from build123d import *

# Parameters (mm, degrees)
SKETCH1_W           = 100
SKETCH1_H           = 70
BOSS_EXTRUDE1_DEPTH = 6.5
SKETCH2_R           = 11.5
CUT_EXTRUDE1_DEPTH  = 19
CUT_EXTRUDE2_DEPTH  = 8
FILLET1_R           = 10


with BuildPart() as part:
    # Sketch1 → Boss-Extrude1 (new body)
    with BuildSketch(Plane(origin=(0, 0, 0), x_dir=(1, 0, 0), z_dir=(0, 1, 0))):
        Rectangle(SKETCH1_W, SKETCH1_H)
    extrude(amount=BOSS_EXTRUDE1_DEPTH)

    # Sketch2 → Cut-Extrude1 (cut)
    with BuildSketch(Plane(origin=(10.212212675, 6.5, 1.842409503), x_dir=(1, 0, 0), z_dir=(0, 1, 0))):
        with Locations((-10.212212675, 1.842409503)):
            Circle(SKETCH2_R)
    extrude(amount=-CUT_EXTRUDE1_DEPTH, mode=Mode.SUBTRACT)

    # Sketch3 → Cut-Extrude2 (cut)
    with BuildSketch(Plane(origin=(10.212212675, 6.5, 1.842409503), x_dir=(1, 0, 0), z_dir=(0, -1, 0))):
        with BuildLine():
            ThreePointArc((-17.21221269, -20.872409503), (-18.202212675, -21.862409519), (-17.212212659, -22.852409503))
            ThreePointArc((-17.212212659, -22.852409503), (-16.222212675, -21.862409488), (-17.21221269, -20.872409503))
        make_face()
        with BuildLine():
            ThreePointArc((-10.212212691, -27.862409503), (-11.212212675, -28.86240952), (-10.212212658, -29.862409503))
            ThreePointArc((-10.212212658, -29.862409503), (-9.212212675, -28.862409487), (-10.212212691, -27.862409503))
        make_face()
        with BuildLine():
            ThreePointArc((-3.212212691, -20.862409503), (-4.212212675, -21.86240952), (-3.212212658, -22.862409503))
            ThreePointArc((-3.212212658, -22.862409503), (-2.212212675, -21.862409487), (-3.212212691, -20.862409503))
        make_face()
    extrude(amount=CUT_EXTRUDE2_DEPTH, mode=Mode.SUBTRACT)

    # Fillet1
    fillet1_edges = [part.edges().sort_by_distance(p)[0] for p in [
        (-50, 3.25, -35),
        (50, 3.25, -35),
        (50, 3.25, 35),
        (-50, 3.25, 35),
    ]]
    fillet(fillet1_edges, radius=FILLET1_R)


solid = part.part
Verification items for the finished model (mm, model axes). Round coordinates to 2 decimals unless told otherwise and drop trailing zeros. Write each loop counter-clockwise with the first axis right and the second up, starting at its lowest first coordinate (ties: lowest second). Pieces come first, ordered by that corner, then holes.
(1) Section check C-C (x = -7). Enter the section's corners in (y, z), plus the area to 3 significant figures.
Returned:
outline: (0, -35) - (6.5, -35) - (6.5, -21.01) - (0, -21.01) - close; (0, -19.03) - (6.5, -19.03) - (6.5, -9.12) - (0, -9.12) - close; (0, 9.12) - (6.5, 9.12) - (6.5, 35) - (0, 35) - close
area: 324 mm2
(2) Mould release check, pull along Z, two halves, no side actions. Record for faces 1 (the flat face through (-12, 0, 0)), 2 (the flat face through (-1, 3, 35)), 3 (the cylindrical face through (-7.602, 3.296, -19.234)): pulls with the +Z half, pulls with the -Z half, needs draft (parallel to the pull), parting line crosses it, or undercut.
Returned:
face 1: needs draft
face 2: pulls with the +Z half
face 3: undercut
(3) Section check D-D (z = -10). Enter the section's corners in (x, y).
Returned:
outline: (-50, 0) - (-5.68, 0) - (-5.68, 6.5) - (-50, 6.5) - close; (5.68, 0) - (50, 0) - (50, 6.5) - (5.68, 6.5) - close
(4) Section check B-B (z = 0). Enter the section's corners in (x, y), plus the area to 4 significant figures.
Returned:
outline: (-50, 0) - (-11.5, 0) - (-11.5, 6.5) - (-50, 6.5) - close; (11.5, 0) - (50, 0) - (50, 6.5) - (11.5, 6.5) - close
area: 500.5 mm2
(5) Section check A-A (y = 4.25). Enter the section's corners in (x, z).
Returned:
outline: (-50, -25) arc R10 ccw to (-40, -35) - (40, -35) arc R10 ccw to (50, -25) - (50, 25) arc R10 ccw to (40, 35) - (-40, 35) arc R10 ccw to (-50, 25) - close; hole circle Ø23 at (0, 0); hole circle Ø1.98 at (-7, -20.02); hole circle Ø2 at (0, -27.02); hole circle Ø2 at (7, -20.02)
(6) Material ranges on line 1 (X direction, y = 1.75, z = -20.02); line 2 (X direction, y = 3.5, z = 0.5); line 3 (X direction, y = 1.5, z = -8.5), recorded low to high.
Returned:
line 1: x = -50 to -7.99, -6.01 to 6, 8 to 50
line 2: x = -50 to -11.49, 11.49 to 50
line 3: x = -50 to -7.75, 7.75 to 50
